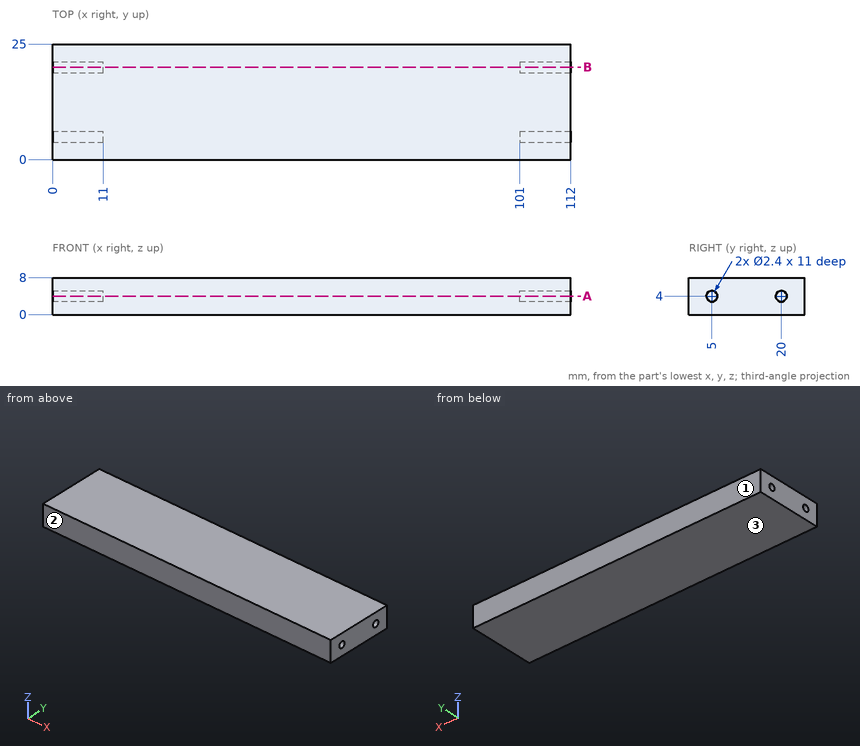
Can you work these out from the drawing? Everything is in mm from the part's minimum corner. Coordinates: 2 decimals unless noted, no trailing zeros. Loops run counter-clockwise (first coordinate to the right, second up) from the corner with the lowest first, then second, coordinate; pieces in that order, holes last.
1. For P1, Ø1.5, axis at y = 14, z = 6.5, coming from the -X side; P2, Ø0.7, axis at y = 20.5, z = 4.5, coming from the -X side; P3, Ø0.7, axis at y = 20, z = 4, coming from the +X side, each with a flat end and sliding along its axis, tell me the tip position at first contact or that it passes through.
2. Imagine slicing it at B-B, the plane y = 20. Please give me the cut outline in (x, z), and give its area (3 significant figures).
3. If we mould it in two halves opening along Y, with no side actions, what happens to the marked faces 1, 2 and 3? For each: pulls with the +Y half, pulls with the -Y half, needs draft (parallel to the pull), parting line crosses it, or undercut.
4. I need wall thicknesses on L1, parallel to Y at x = 107, z = 4; L2, parallel to Z at x = 5.5, y = 5; L3, parallel to X at y = 19.25, z = 4.75. Which ranges of each line are inside material? Lowest first, please.
5. Imagine slicing it at A-A, the plane z = 4. Please give me the cut outline in (x, y), and give its area (3 significant figures).
Taken from the geometry:
1. P1: stops at x = 0
1. P2: stops at x = 11
1. P3: stops at x = 101
2. outline: (0, 0) - (112, 0) - (112, 2.8) - (101, 2.8) - (101, 5.2) - (112, 5.2) - (112, 8) - (0, 8) - (0, 5.2) - (11, 5.2) - (11, 2.8) - (0, 2.8) - close
2. area: 843 mm2
3. face 1: pulls with the +Y half
3. face 2: pulls with the -Y half
3. face 3: needs draft
4. L1: y = 0 to 3.8, 6.2 to 18.8, 21.2 to 25
4. L2: z = 0 to 2.8, 5.2 to 8
4. L3: x = 11 to 101
5. outline: (0, 0) - (112, 0) - (112, 3.8) - (101, 3.8) - (101, 6.2) - (112, 6.2) - (112, 18.8) - (101, 18.8) - (101, 21.2) - (112, 21.2) - (112, 25) - (0, 25) - (0, 21.2) - (11, 21.2) - (11, 18.8) - (0, 18.8) - (0, 6.2) - (11, 6.2) - (11, 3.8) - (0, 3.8) - close
5. area: 2,690 mm2
